Geometry: final body of the model. Coordinates: model frame, mm. A direction names the side the tool comes from. Give positions to 0.01 mm unless a question says otherwise; leave off trailing zeros. Loops run counter-clockwise (first coordinate to the right, second up) from the corner with the lowest first, then second, coordinate; pieces in that order, holes last.
```python
from build123d import *

# Parameters (mm, degrees)
SKETCH_1_R      = 2.05
SKETCH_1_R_2    = 5.025
SKETCH_1_R_3    = 1.65
SKETCH_1_W      = 2.1
SKETCH_1_H      = 8.1
EXTRUDE_1_DEPTH = 2
FILLET_1_R      = 1.3
FILLET_2_R      = 2
FILLET_3_R      = 5


with BuildPart() as part:
    # 草图1 → 凸台-拉伸1 (new body)
    with BuildSketch(Plane.XY):
        with BuildLine():
            Line((32.115707856, 28), (32.115707856, 22.85))
            Line((32.115707856, 22.85), (30.015707856, 22.85))
            Line((30.015707856, 22.85), (30.015707856, 28))
            Line((30.015707856, 28), (-29.075, 28))
            Line((-29.075, 28), (-38.998995168, 22.002009663))
            ThreePointArc((-38.998995168, 22.002009663), (-52.370174504, 17.472835843), (-60.236366221, 5.75))
            Line((-60.236366221, 5.75), (-79.631279411, 5.75))
            Line((-79.631279411, 5.75), (-79.631279411, -5.75))
            Line((-79.631279411, -5.75), (-60.236366221, -5.75))
            ThreePointArc((-60.236366221, -5.75), (-52.370174504, -17.472835843), (-38.998995168, -22.002009663))
            Line((-38.998995168, -22.002009663), (-29.075, -28))
            Line((-29.075, -28), (30.015707856, -28))
            Line((30.015707856, -28), (30.015707856, -22.85))
            Line((30.015707856, -22.85), (32.115707856, -22.85))
            Line((32.115707856, -22.85), (32.115707856, -28))
            Line((32.115707856, -28), (36.001004832, -41.401911511))
            Line((36.001004832, -41.401911511), (73.077470353, -41.401911511))
            Line((73.077470353, -41.401911511), (73.077470353, -21.401911511))
            Line((73.077470353, -21.401911511), (36.001004832, -21.401911511))
            Line((36.001004832, -21.401911511), (36.001004832, 28))
            Line((36.001004832, 28), (32.115707856, 28))
        make_face()
        with Locations((31.065707856, 15)):
            Circle(SKETCH_1_R, mode=Mode.SUBTRACT)
        with Locations(Location((31.065707856, -15, 0), (0, 0, 180))):
            Circle(SKETCH_1_R, mode=Mode.SUBTRACT)
        with Locations((-38.998995168, 0)):
            Circle(SKETCH_1_R_2, mode=Mode.SUBTRACT)
        with Locations((1.001004832, -25)):
            Circle(SKETCH_1_R, mode=Mode.SUBTRACT)
        with Locations((1.001004832, 25)):
            Circle(SKETCH_1_R, mode=Mode.SUBTRACT)
        with Locations((-74.958287312, 0)):
            Circle(SKETCH_1_R, mode=Mode.SUBTRACT)
        with Locations((-50.998995168, 0)):
            Circle(SKETCH_1_R_3, mode=Mode.SUBTRACT)
        with Locations((-38.998995168, 12)):
            Circle(SKETCH_1_R_3, mode=Mode.SUBTRACT)
        with Locations((-26.998995168, 0)):
            Circle(SKETCH_1_R_3, mode=Mode.SUBTRACT)
        with Locations((-38.998995168, -12)):
            Circle(SKETCH_1_R_3, mode=Mode.SUBTRACT)
        with Locations((31.065707856, 0)):
            Rectangle(SKETCH_1_W, SKETCH_1_H, mode=Mode.SUBTRACT)
        Polygon((2.100885183, -16.20323489), (23.065707856, -9.230000311), (23.065707856, 9.230000311), (2.100885183, 16.20323489), (-21.039703025, 1.3748119), (-21.039703025, -1.3748119), align=None, mode=Mode.SUBTRACT)
        with BuildLine():
            Line((55.751004832, -35.401911511), (55.751004832, -27.401911511))
            ThreePointArc((55.751004832, -27.401911511), (57.001004832, -26.151911511), (58.251004832, -27.401911511))
            Line((58.251004832, -27.401911511), (58.251004832, -35.401911511))
            ThreePointArc((58.251004832, -35.401911511), (57.001004832, -36.651911511), (55.751004832, -35.401911511))
        make_face(mode=Mode.SUBTRACT)
        with BuildLine():
            Line((67.751004832, -27.401911511), (67.751004832, -35.401911511))
            ThreePointArc((67.751004832, -35.401911511), (66.501004832, -36.651911511), (65.251004832, -35.401911511))
            Line((65.251004832, -35.401911511), (65.251004832, -27.401911511))
            ThreePointArc((65.251004832, -27.401911511), (66.501004832, -26.151911511), (67.751004832, -27.401911511))
        make_face(mode=Mode.SUBTRACT)
    extrude(amount=EXTRUDE_1_DEPTH)

    # 圆角1
    fillet_1_edges = [part.edges().sort_by_distance(p)[0] for p in [
        (-60.236366221, -5.75, 1),
        (-79.631279411, -5.75, 1),
        (-79.631279411, 5.75, 1),
        (-60.236366221, 5.75, 1),
        (30.015707856, 28, 1),
        (32.115707856, 28, 1),
        (30.015707856, -28, 1),
    ]]
    fillet(fillet_1_edges, radius=FILLET_1_R)

    # 圆角2
    fillet_2_edges = [part.edges().sort_by_distance(p)[0] for p in [
        (2.100885183, -16.20323489, 1),
        (23.065707856, -9.230000311, 1),
        (23.065707856, 9.230000311, 1),
        (2.100885183, 16.20323489, 1),
        (-21.039703025, 1.3748119, 1),
        (-21.039703025, -1.3748119, 1),
    ]]
    fillet(fillet_2_edges, radius=FILLET_2_R)

    # 圆角3
    fillet_3_edges = [part.edges().sort_by_distance(p)[0] for p in [
        (36.001004832, -21.401911511, 1),
    ]]
    fillet(fillet_3_edges, radius=FILLET_3_R)


solid = part.part
```
Q1. Mould query, pull axis X, two halves, no side actions, for faces 1 (the face through (37.43, -19.9, 1.01)), 2 (the face through (-73, 0.6, 1)), 3 (the face through (34.03, -34.61, 0.99)). Classes: +X half, -X half, draft (parallel to the pull), parting line (faces both ways), or undercut.
Q2. Section query C-C, the plane z = 0.9. State how many separate pieces and enclosed holes the cut face has, and give its area (3 significant figures).
Q3. Section query B-B, the plane y = 25. Return loops of the section in (x, z).
Q4. Material intervals for probe 1 along Y at (x, z) = (2.5, 0.2); probe 2 along X at (y, z) = (-5.5, 1.95); probe 3 along Y at (x, z) = (26, 1.8), sorted ascending.
Q5. Reachability of faces 4 (the face through (-4, -14, 0)), 5 (the face through (-9.261, 8.923, 0.986)) from +Z, -Z, +X, -X, +Y, -Y: full face, straight path, thin tool, end or side. Return the list, or none.
Q6. Pin query (flat end, axial travel): pin 1 Ø1 at (y, z) = (9.5, 1) entering from +X; pin 2 Ø0.6 at (x, z) = (30.5, 0.5) entering from +Y; pin 3 Ø0.6 at (x, z) = (-70, 1) entering from -Y. Return the tip coordinate at first contact, or that it passes through.
Q7. Section query A-A, the plane x = 9. Return loops of the section in (y, z).
Resolved:
1. face 1: +X half
1. face 2: undercut
1. face 3: -X half
2. separate pieces: 1
2. enclosed holes: 14
2. area: 4,680 mm2
3. outline: (-34.04, 0) - (-1.05, 0) - (-1.05, 2) - (-34.04, 2) - close; (3.05, 0) - (30.02, 0) - (30.02, 2) - (3.05, 2) - close; (32.12, 0) - (36, 0) - (36, 2) - (32.12, 2) - close
4. probe 1: y = -28 to -26.4, -23.6 to -16, 16 to 23.6, 26.4 to 28
4. probe 2: x = -79.1 to -14.6, 23.07 to 36
4. probe 3: y = -28 to 28
5. face 4: -Z, +X, -X, +Y, -Y
5. face 5: +Z, -Z
6. pin 1: stops at x = 36
6. pin 2: stops at y = 22.85
6. pin 3: stops at y = -5.75
7. outline: (-28, 0) - (-13.91, 0) - (-13.91, 2) - (-28, 2) - close; (13.91, 0) - (28, 0) - (28, 2) - (13.91, 2) - close
